The model under review builds one solid part; all positions refer to its coordinate system, in mm. A direction names the side the tool comes from. Coordinates: 2 decimals unless noted, no trailing zeros. Order: outer loops, then holes, each group sorted by start corner. A loop starts at its lowest first (then second) coordinate and runs counter-clockwise, first axis right, second up. Notation, with made-up numbers: (-21.75, 65) -> (-8.75, 65) arc R28 cw to (-8.75, 85) -> close; hole circle Ø2 at (79.25, 74). An arc over 180 degrees is marked (long way). Put each result on its own line as item: value.
from build123d import *

# Parameters (mm, degrees)
BOSS_EXTRUDE1_DEPTH = 9.6
SKETCH2_R           = 2.4
BOSS_EXTRUDE2_DEPTH = 1.6
LPATTERN1_COUNT     = 3
LPATTERN1_PITCH     = 8
SHELL1_T            = -1.6
SKETCH3_R           = 2.4
CUT_EXTRUDE1_DEPTH  = 1.6


with BuildPart() as part:
    # Sketch1 → Boss-Extrude1 (new body)
    with BuildSketch(Plane(origin=(0, 0, 0), x_dir=(1, 0, 0), z_dir=(0, 1, 0))):
        Polygon((0, 0), (-8, 0), (-16, 24), (0, 24), align=None)
    extrude(amount=BOSS_EXTRUDE1_DEPTH)

    # Sketch2 → Boss-Extrude2 (add)
    with BuildSketch(Plane(origin=(0, 9.6, 0), x_dir=(1, 0, 0), z_dir=(0, 1, 0))):
        with Locations(Location((-4, 4, 0), (0, 0, 90))):
            Circle(SKETCH2_R)
    boss_extrude2 = extrude(amount=BOSS_EXTRUDE2_DEPTH)

    # LPattern1: Boss-Extrude2 ×3
    with Locations(*[(0, 0, -i * LPATTERN1_PITCH) for i in range(1, LPATTERN1_COUNT)]):
        add(boss_extrude2)

    # Shell1
    shell1_openings = [part.faces().sort_by_distance(p)[0] for p in [
        (-6.222222222, 0, -13.333333333),
    ]]
    offset(amount=SHELL1_T, openings=shell1_openings, kind=Kind.INTERSECTION)

    # Sketch3 → Cut-Extrude1 (cut)
    with BuildSketch(Plane.XZ):
        with Locations((-12, -12)):
            Circle(SKETCH3_R)
        with Locations((-12, -20)):
            Circle(SKETCH3_R)
    extrude(amount=-CUT_EXTRUDE1_DEPTH, mode=Mode.SUBTRACT)


solid = part.part
Item 1: Consider section C-C on y = 5.75. Write out the cut boundary in (x, z).
Answers below:
outline: (-16, -24) -> (0, -24) -> (0, 0) -> (-8, 0) -> close; hole (-13.78, -22.4) -> (-1.6, -22.4) -> (-1.6, -1.6) -> (-6.85, -1.6) -> close
Item 2: For pin 1 Ø2 at (y, z) = (5, -21.5) entering from -X; pin 2 Ø4 at (x, z) = (-13, -10) entering from +Y; pin 3 Ø4 at (y, z) = (5.5, -16) entering from -X; pin 4 Ø8 at (x, z) = (-8, -10.5) entering from +Y, all flat-tipped, find the tip position at first contact; note any pin that passes through.
Answers below:
pin 1: x = -15.5
pin 2: y = 9.6
pin 3: x = -14
pin 4: y = 11.2
Item 3: For faces 1 (the cylindrical face through (-6.024, 10.389, -13.29)), 2 (the flat face through (-6, 8, -14)), 3 (the cylindrical face through (-10.47, 0.79, -10.15)), list the 3-axis set-ups (+Z, -Z, +X, -X, +Y, -Y) from which the entire face can be reached by the end or side of a thin tool; tool diameter is ignored.
Answers below:
face 1: +Y
face 2: -Y
face 3: -X, -Y
Item 4: Consider section A-A on y = 8.25. Write out the cut boundary in (x, z).
Answers below:
outline: (-16, -24) -> (0, -24) -> (0, 0) -> (-8, 0) -> close; hole circle Ø1.6 at (-4, -20); hole circle Ø1.6 at (-4, -12); hole circle Ø1.6 at (-4, -4)
Item 5: For line 1 (Z direction, x = -6, y = 6.75); line 2 (Y direction, x = -0.5, z = -5.75); line 3 (Y direction, x = -4.75, z = -7.25), list the stretches that pass through material, from the lowest coordinate up. Write a range as from..to.
Answers below:
line 1: -24..-22.4, -1.6..0
line 2: 0..9.6
line 3: 8..9.6
Item 6: Consider section D-D on z = -18.5. Write out the cut boundary in (x, y).
Answers below:
outline: (-14.17, 0) -> (-13.87, 0) -> (-13.87, 1.6) -> (-12.48, 1.6) -> (-12.48, 8) -> (-1.6, 8) -> (-1.6, 0) -> (0, 0) -> (0, 9.6) -> (-2.13, 9.6) -> (-2.13, 11.2) -> (-5.87, 11.2) -> (-5.87, 9.6) -> (-14.17, 9.6) -> close
Item 7: Mouldability with a two-part tool opening along Z and no side actions: class faces 4 (the flat face through (-4, 11.2, -12)), 5 (the cylindrical face through (-4.106, 10.389, -17.602)) as +Z half, -Z half, draft (parallel to the pull), parting line (faces both ways), or undercut.
Answers below:
face 4: draft
face 5: undercut
